The listing builds one solid part. Answer for the finished solid, in the listing's coordinates (mm). Round coordinates to 2 decimals unless told otherwise and drop trailing zeros. Write each loop counter-clockwise with the first axis right and the second up, starting at its lowest first coordinate (ties: lowest second). Pieces come first, ordered by that corner, then holes. Notation, with made-up numbers: M -15,15.25 L 28,15.25 A21 cw 28,41.25 Z; hole C 1,32.5 d7. An arc over 180 degrees is marked long. One line per item, written item: value. Start each with the question number.
(1) Consider probe 1 along Z at (x, y) = (3.45, 0); probe 2 along Y at (x, z) = (0.8, 1.5); probe 3 along Y at (x, z) = (3.5, -2.25). Determine where each line is inside the solid, lowest interval first.
(2) Given P1, Ø5.5, axis at y = 0, z = 0, coming from the -X side; P2, Ø1.5, axis at x = 1, z = -1, coming from the -Y side; P3, Ø2, axis at x = 4, z = 1.5, coming from the +Y side, each flat-ended and moving along its own axis, determine where each tip first touches the part or whether it passes through.
(3) For a pull along Y with two mould halves and no side action, classify faces 1 (the flat face through (2.47, 4.31, 2.535)), 2 (the cylindrical face through (2.469, -0.738, -2.345)), 3 (the flat face through (2, 0, -5)) as released by +Y, released by -Y, zero draft, split by the parting line, or undercut.
(4) Section A-A (y = 0) is taken. Determine the outline of the cut face in (x, z), plus the area to 3 significant figures.
(5) Section B-B (x = 2.5) is taken. Determine the outline of the cut face in (y, z), plus the area to 3 significant figures.
(6) Section C-C (x = 0.6) is taken. Determine the outline of the cut face in (y, z), plus the area to 3 significant figures.
Autodesk Inventor part; units mm, degrees
ref_plane "Work Plane1" through (-11.098, 0, 0) normal (0, -0.8660254, -0.5) x (1, 0, 0)
ref_plane "YZ Plane" through (0, 0, 0) normal (1, 0, 0) x (0, 1, 0)
ref_plane "XZ Plane" through (0, 0, 0) normal (0, 1, 0) x (-1, 0, 0)
sketch "Sketch1" plane through (0, 0, 0) normal (1, 0, 0) x (0, 1, 0)
  line L0 (-5.7735, 0) -> (-2.8868, 5)
  line L1 (-2.8868, 5) -> (2.8868, 5)
  line L2 (2.8868, 5) -> (5.7735, 0)
  line L3 (5.7735, 0) -> (2.8868, -5)
  line L4 (2.8868, -5) -> (-2.8868, -5)
  line L5 (-2.8868, -5) -> (-5.7735, 0)
  point P0 (0, 0)
  point P1 (0, 0)
  dimension "d0" = 11.547
extrude "Body" add sketch "Sketch1" along normal blind 5
sketch "Sketch2" plane through (0, 0, 0) normal (0, 0, 1) x (1, 0, 0)
  line L0 (0, 2.8868) -> (0, 5.7735)
  line L1 (0, 5.7735) -> (5, 5.7735)
  line L2 (5, 2.8868) -> (5, 5.7735)
  line L3 (-1, 0) -> (6, 0)
  line L4 (0.793, 5.7735) -> (0, 4.4)
  line L5 (4.207, 5.7735) -> (5, 4.4)
  dimension "d3" = 30
  dimension "d4" = 30
  dimension "d5" = 8.8
  dimension "d6" = 8.8
revolve "Chamfer1" cut sketch "Sketch2" angle 360 about axis through (-10, 0, 0) along (1, 0, 0)
sketch "Sketch3" plane through (5, 0, 0) normal (1, 0, 0) x (0, 0, -1)
  arc A0 (-0.625, -1.0825) -> (0.625, -1.0825) centre (0, 0) ccw
hole "Thread" at (5, 0, 0) direction (-1, 0, 0) diameter 4.917 end through all
chamfer "Chamfer2" distance 0.5413 angle 30 1 edges at (5, 0, 2.4585) measured on face at (5, 3.7042, -0.4498)
chamfer "Chamfer3" distance 0.5413 angle 30 1 edges at (0, 0, 2.4585) measured on face at (0, 3.7042, -0.4498)
ref_plane "Work Plane1" through (-11.098, 0, 0) normal (0, -0.8660254, -0.5) x (1, 0, 0)
equation "\"d0\" = 1.1547 * SW"
equation "\"d1\" = KOH"
equation "\"d8\" = -0.5 * GD1 + 0.5 * NND"
equation "\"d40\" = -0.5 * GD1 + 0.5 * NND"
equation "\"d10\" = -0.5 * GD1 + 0.5 * NND"
equation "\"d41\" = -0.5 * GD1 + 0.5 * NND"
equation "\"d3\" = ANG1"
equation "\"d4\" = ANG2"
equation "\"d5\" = SW0"
equation "\"d6\" = SW01"
equation "\"ANG1\" = 30deg"
equation "\"ANG2\" = 30deg"
equation "\"NND\" = 6"
equation "\"KOH\" = 5"
equation "\"SW0\" = SW01"
equation "\"SW01\" = 8.8"
equation "\"GUL\" = 0.541266 * PTC"
equation "\"THREADDIA\" = 6"
equation "\"TOA\" = 30deg"
equation "\"PTC\" = 1"
equation "\"E0\" = 1.155 * SW"
equation "\"GAL\" = 0.541266 * PTC"
properties part number "DIN 934 - M6" material "Steel, Mild"
Recorded:
1. probe 1: z = -5 to -2.46, 2.46 to 5
1. probe 2: y = -4.91 to -1.95, 1.95 to 4.91
1. probe 3: y = -4.47 to -0.99, 0.99 to 4.47
2. P1: stops at x = 0.14
2. P2: stops at y = -5.63
2. P3: stops at y = 5.48
3. face 1: released by +Y
3. face 2: undercut
3. face 3: zero draft
4. outline: M 0,-4.4 L 0.35,-5 L 4.65,-5 L 5,-4.4 L 5,-3 L 4.69,-2.46 L 0.31,-2.46 L 0,-3 Z; M 0,3 L 0.31,2.46 L 4.69,2.46 L 5,3 L 5,4.4 L 4.65,5 L 0.35,5 L 0,4.4 Z
4. area: 24.7 mm2
5. outline: M -5.77,0 L -2.89,-5 L 2.89,-5 L 5.77,0 L 2.89,5 L -2.89,5 Z; hole C 0,0 d4.92
5. area: 67.6 mm2
6. outline: M -5.4,-0.65 L -3.26,-4.35 A5.44 ccw -2.14,-5 L 2.14,-5 A5.44 ccw 3.26,-4.35 L 5.4,-0.65 A5.44 ccw 5.4,0.65 L 3.26,4.35 A5.44 ccw 2.14,5 L -2.14,5 A5.44 ccw -3.26,4.35 L -5.4,0.65 A5.44 ccw Z; hole C 0,0 d4.92
6. area: 66.4 mm2
